```python
from build123d import *

# Parameters (mm, degrees)
SKETCH_1_R           = 1.5
EXTRUDE_1_DEPTH      = 3
SKETCH_2_R           = 2.5
SKETCH_2_R_2         = 1.5
EXTRUDE_2_DEPTH      = 15
SKETCH_3_W           = 5
SKETCH_3_H           = 3
EXTRUDE_3_DEPTH      = 35.032354187
EXTRUDE_4_DEPTH      = 5
SKETCH_5_R           = 12.5
SKETCH_5_R_2         = 7.5
EXTRUDE_5_DEPTH      = 1
SKETCH_6_R           = 12.5
SKETCH_6_R_2         = 11.1
EXTRUDE_6_DEPTH      = 5
EXTRUDE_7_DEPTH      = 5
EXTRUDE_7_DEPTH_BACK = 1
CHAMFER_1_SIZE       = 5
FILLET_1_R           = 2


with BuildPart() as part:
    # Sketch 1 → Extrude 1 (new body)
    with BuildSketch(Plane(origin=(0, 0, 0), x_dir=(1, 0, 0), z_dir=(0, 1, 0))):
        with BuildLine():
            Line((-6.310049273, -9.865580478), (0, -3.539912271))
            Line((0, -3.539912271), (6.310049273, -9.865580478))
            ThreePointArc((6.310049273, -9.865580478), (9.845580478, -9.869950727), (9.849950727, -6.334419522))
            Line((9.849950727, -6.334419522), (3.531171747, 0))
            Line((3.531171747, 0), (9.849950727, 6.334419522))
            ThreePointArc((9.849950727, 6.334419522), (9.845580478, 9.869950727), (6.310049273, 9.865580478))
            Line((6.310049273, 9.865580478), (2.5, 6.04610039))
            Line((2.5, 6.04610039), (2.5, 26.04610039))
            Line((2.5, 26.04610039), (-2.5, 26.04610039))
            Line((-2.5, 26.04610039), (-2.5, 6.04610039))
            Line((-2.5, 6.04610039), (-6.310049273, 9.865580478))
            ThreePointArc((-6.310049273, 9.865580478), (-9.845580478, 9.869950727), (-9.849950727, 6.334419522))
            Line((-9.849950727, 6.334419522), (-3.531171747, 0))
            Line((-3.531171747, 0), (-9.849950727, -6.334419522))
            ThreePointArc((-9.849950727, -6.334419522), (-9.845580478, -9.869950727), (-6.310049273, -9.865580478))
        make_face()
        with Locations(Location((-8.08, 8.1, 0), (0, 0, 270))):
            Circle(SKETCH_1_R, mode=Mode.SUBTRACT)
        with Locations(Location((8.08, 8.1, 0), (0, 0, 270))):
            Circle(SKETCH_1_R, mode=Mode.SUBTRACT)
        with Locations(Location((-8.08, -8.1, 0), (0, 0, 270))):
            Circle(SKETCH_1_R, mode=Mode.SUBTRACT)
        with Locations(Location((8.08, -8.1, 0), (0, 0, 270))):
            Circle(SKETCH_1_R, mode=Mode.SUBTRACT)
    extrude(amount=EXTRUDE_1_DEPTH)

    # Sketch 2 → Extrude 2 (add)
    # profile 1 of 4: a face of its own
    with BuildSketch(Plane(origin=(0, 3, 0), x_dir=(1, 0, 0), z_dir=(0, 1, 0))):
        with Locations(Location((-8.08, -8.1, 0), (0, 0, 135.07082293))):
            Circle(SKETCH_2_R)
        with Locations(Location((-8.08, -8.1, 0), (0, 0, 270))):
            Circle(SKETCH_2_R_2, mode=Mode.SUBTRACT)
    # profile 2 of 4: a face of its own
    with BuildSketch(Plane(origin=(0, 3, 0), x_dir=(1, 0, 0), z_dir=(0, 1, 0))):
        with Locations(Location((-8.08, 8.1, 0), (0, 0, 44.92917707))):
            Circle(SKETCH_2_R)
        with Locations(Location((-8.08, 8.1, 0), (0, 0, 270))):
            Circle(SKETCH_2_R_2, mode=Mode.SUBTRACT)
    # profile 3 of 4: a face of its own
    with BuildSketch(Plane(origin=(0, 3, 0), x_dir=(1, 0, 0), z_dir=(0, 1, 0))):
        with Locations(Location((8.08, 8.1, 0), (0, 0, 135.07082293))):
            Circle(SKETCH_2_R)
        with Locations(Location((8.08, 8.1, 0), (0, 0, 270))):
            Circle(SKETCH_2_R_2, mode=Mode.SUBTRACT)
    # profile 4 of 4: a face of its own
    with BuildSketch(Plane(origin=(0, 3, 0), x_dir=(1, 0, 0), z_dir=(0, 1, 0))):
        with Locations(Location((8.08, -8.1, 0), (0, 0, 44.92917707))):
            Circle(SKETCH_2_R)
        with Locations(Location((8.08, -8.1, 0), (0, 0, 270))):
            Circle(SKETCH_2_R_2, mode=Mode.SUBTRACT)
    extrude(amount=EXTRUDE_2_DEPTH)

    # Sketch 3 → Extrude 3 (add)
    with BuildSketch(Plane(origin=(0, 3, 0), x_dir=(1, 0, 0), z_dir=(0, 1, 0))):
        with Locations((0, 14.54610039)):
            Rectangle(SKETCH_3_W, SKETCH_3_H)
    extrude(amount=EXTRUDE_3_DEPTH)

    # Sketch 4 → Extrude 4 (add)
    with BuildSketch(Plane(origin=(2.5, 0, 0), x_dir=(0, 0, -1), z_dir=(1, 0, 0))):
        Polygon((16.04610039, 38.032354187), (26.04610039, 3), (22.926270675, 3), (16.04610039, 27.10285623), align=None)
    extrude(amount=-EXTRUDE_4_DEPTH)



with BuildPart() as body_2:
    # Sketch 5 → Extrude 5 (new body)
    with BuildSketch(Plane(origin=(0, 38.032354187, 0), x_dir=(1, 0, 0), z_dir=(0, 1, 0))):
        with Locations(Location((0, 0, 0), (0, 0, 270))):
            Circle(SKETCH_5_R)
        with Locations(Location((0, 0, 0), (0, 0, 270))):
            Circle(SKETCH_5_R_2, mode=Mode.SUBTRACT)
    extrude(amount=-EXTRUDE_5_DEPTH)

    # Sketch 6 → Extrude 6 (add)
    with BuildSketch(Plane(origin=(0, 38.032354187, 0), x_dir=(1, 0, 0), z_dir=(0, 1, 0))):
        with Locations(Location((0, 0, 0), (0, 0, 270))):
            Circle(SKETCH_6_R)
        with Locations(Location((0, 0, 0), (0, 0, 270))):
            Circle(SKETCH_6_R_2, mode=Mode.SUBTRACT)
    extrude(amount=EXTRUDE_6_DEPTH)


with BuildPart() as part_1:
    add(part.part)

    add(body_2.part)  # Extrude 7 merges body 2
    # Sketch 7 → Extrude 7 (add, two sides: drawn at the far end of the back side and taken through both)
    with BuildSketch(Plane(origin=(0, 38.032354187, 0), x_dir=(1, 0, 0), z_dir=(0, 1, 0)).offset(-EXTRUDE_7_DEPTH_BACK)):
        with BuildLine():
            Line((-2.5, 16.04610039), (2.5, 16.04610039))
            Line((2.5, 16.04610039), (2.5, 12.247448714))
            ThreePointArc((2.5, 12.247448714), (0, 12.5), (-2.5, 12.247448714))
            Line((-2.5, 12.247448714), (-2.5, 16.04610039))
        make_face()
    extrude(amount=EXTRUDE_7_DEPTH + EXTRUDE_7_DEPTH_BACK)

    # Chamfer 1
    chamfer_1_edges = [part_1.edges().sort_by_distance(p)[0] for p in [
        (0, 37.032354187, -13.04610039),
    ]]
    chamfer(chamfer_1_edges, length=CHAMFER_1_SIZE)

    # Fillet 1
    fillet_1_edges = [part_1.edges().sort_by_distance(p)[0] for p in [
        (-3.531171747, 1.5, 0),
        (-2.5, 1.5, -6.04610039),
        (-2.5, 1.5, -26.04610039),
        (2.5, 1.5, -26.04610039),
        (2.5, 1.5, -6.04610039),
        (3.531171747, 1.5, 0),
        (0, 1.5, 3.539912271),
    ]]
    fillet(fillet_1_edges, radius=FILLET_1_R)


solid = part_1.part
```
Input: part model. Units: mm. Frame: model coordinates. A direction names the side the tool comes from. Round coordinates to 2 decimals unless told otherwise and drop trailing zeros. Loops run counter-clockwise (first coordinate to the right, second up) from the corner with the lowest first, then second, coordinate; pieces in that order, holes last. Notation, with made-up numbers: (-21, 21.5) - (15, 21.5) arc R34 ccw to (15, 55.5) - close; hole circle Ø8 at (75, -31). An arc over 180 degrees is marked (long way). One line per item, written item: value. Start each with the question number.
(1) Section A-A, the plane z = 0. Return loops of the section in (x, y), plus the area to 3 significant figures.
(2) Contact query for flat-ended pins moving along their axis: P1, Ø4, axis at x = 4, y = 21.5, coming from the +Z side; P2, Ø10, axis at x = -1.5, z = -0.5, coming from the -Y side; P3, Ø1.5, axis at x = 1, y = 12, coming from the -Z side; P4, Ø1.5, axis at x = -3, y = 20, coming from the -Z side. Output: stop coordinate, or through.
(3) Access query for faces 5 (the flat face through (0, 17, -13.046)), 6 (the cylindrical face through (8.53, 8.87, 9.53)), 7 (the flat face through (0.035, 14.883, -19.534)), 8 (the flat face through (10, 18, 8)), 9 (the cylindrical face through (0.33, 37.539, -7.493)). Directions: +Z, -Z, +X, -X, +Y, -Y. A direction counts if a zero-diameter tool reaches every point of the face in a straight line with its end or side. Return the directions, or none.
(4) Section C-C, the plane z = 8.1. Return loops of the section in (x, y).
(5) Section B-B, the plane y = 6. Count the separate pieces of the cut face and the enclosed holes in it, plus the area to 3 significant figures.
(6) Draft query along X for faces 1 (the flat face through (3.83, 1.48, 7.38)), 2 (the flat face through (7.36, 1.48, -3.84)), 3 (the cylindrical face through (3.705, 1.521, -9.048)), 4 (the flat face through (0, 3, -20)). Return one class per face: +X half, -X half, draft (parallel to the pull), parting line (faces both ways), or undercut.
(7) Section D-D, the plane y = 22. Return loops of the section in (x, z).
(8) Ray query, line 1 (X direction, y = 11.25, z = -8.1); line 2 (Y direction, x = 10.5, z = -8.5); line 3 (X direction, y = 35.5, z = -15). Return the intervals inside material, ascending. Write a range as [from, to].
Results below:
1. outline: (-12.5, 37.03) - (-7.5, 37.03) - (-7.5, 38.03) - (-11.1, 38.03) - (-11.1, 43.03) - (-12.5, 43.03) - close; (-4.36, 0) - (4.36, 0) - (4.36, 3) - (-4.36, 3) - close; (7.5, 37.03) - (12.5, 37.03) - (12.5, 43.03) - (11.1, 43.03) - (11.1, 38.03) - (7.5, 38.03) - close
1. area: 50.1 mm^2
2. P1: z = -13.05
2. P2: y = 0
2. P3: z = -23.69
2. P4: z = -21.35
3. face 5: +Z, +X, -X
3. face 6: -Y
3. face 7: +X, -X
3. face 8: +Z, -Z, +X, -X
3. face 9: +Y
4. outline: (-10.58, 0) - (-9.58, 0) - (-9.58, 18) - (-10.58, 18) - close; (-9.52, 37.03) - (9.52, 37.03) - (9.52, 43.03) - (7.59, 43.03) - (7.59, 38.03) - (-7.59, 38.03) - (-7.59, 43.03) - (-9.52, 43.03) - close; (-6.58, 0) - (-4.55, 0) - (-4.55, 3) - (-5.58, 3) - (-5.58, 18) - (-6.58, 18) - close; (4.55, 0) - (6.58, 0) - (6.58, 18) - (5.58, 18) - (5.58, 3) - (4.55, 3) - close; (9.58, 0) - (10.58, 0) - (10.58, 18) - (9.58, 18) - close
5. separate pieces: 6
5. enclosed holes: 4
5. area: 80.6 mm^2
6. face 1: undercut
6. face 2: +X half
6. face 3: undercut
6. face 4: draft
7. outline: (-2.5, -20.62) - (2.5, -20.62) - (2.5, -17.5) - (-2.5, -17.5) - close; (-2.5, -16.05) - (2.5, -16.05) - (2.5, -13.05) - (-2.5, -13.05) - close
8. line 1: [-10.58, -9.58], [-6.58, -5.58], [5.58, 6.58], [9.58, 10.58]
8. line 2: [0, 18]
8. line 3: [-2.5, 2.5]
